The model under review builds one solid part; all positions refer to its coordinate system, in mm. Round coordinates to 2 decimals unless told otherwise and drop trailing zeros. Loops run counter-clockwise (first coordinate to the right, second up) from the corner with the lowest first, then second, coordinate; pieces in that order, holes last. Notation, with made-up numbers: M 11,21 L 56,21 A22 ccw 56,29 Z; hole C 36,68 d11. An arc over 180 degrees is marked long. Answer in a Markdown table with one row per item. Add a question column.
Autodesk Inventor part; units mm, degrees
ref_plane "YZ Plane" through (0, 0, 0) normal (1, 0, 0) x (0, 1, 0)
ref_plane "XZ Plane" through (0, 0, 0) normal (0, 1, 0) x (-1, 0, 0)
ref_plane "XY Plane" through (0, 0, 0) normal (0, 0, 1) x (1, 0, 0)
sketch "Sketch1" plane through (0, 0, 0) normal (0, 0, 1) x (1, 0, 0)
  circle A0 centre (0, 0) radius 47.625
  dimension "d0" = 95.25
extrude "Extrusion1" add sketch "Sketch1" along normal blind 3.175
sketch "Sketch4" plane through (0, 0, 3.175) normal (0, 0, 1) x (1, 0, 0)
  circle A0 centre (12.446, -29.7561) radius 3.3655
  point P0 (0, 0)
  dimension "d16" = 6.731
  dimension "d17" = 12.446
  dimension "d18" = 29.7561
extrude "Extrusion4" cut sketch "Sketch4" against normal blind 3.175
sketch "Sketch6" plane through (0, 0, 3.175) normal (0, 0, 1) x (1, 0, 0)
  circle A0 centre (0, 0) radius 3.3655
  circle A1 centre (0, 0) radius 9.525
  circle A2 centre (0, 0) radius 47.625
  circle A3 centre (12.446, -29.7561) radius 3.3655
  line L0 (0, 0) -> (12.446, -29.7561) construction
  dimension "d32" = 6.731
  dimension "d33" = 19.05
  dimension "d191" = 32.2541
extrude "Extrusion7" add sketch "Sketch6" along normal blind 3.81 contours A1
sketch "Sketch7" plane through (0, 0, 3.175) normal (0, 0, 1) x (1, 0, 0)
  line L0 (0, 0) -> (21.4313, 37.12)
  line L1 (0, 0) -> (42.8625, 0) construction
  circle A0 centre (21.4313, 37.12) radius 1.8415
  circle A1 centre (-21.4312, 37.12) radius 1.8415
  circle A2 centre (-42.8625, 0) radius 1.8415
  circle A3 centre (-21.4313, -37.12) radius 1.8415
  circle A4 centre (21.4312, -37.12) radius 1.8415
  circle A5 centre (42.8625, 0) radius 1.8415
  dimension "d39" = 42.8625
  dimension "d40" = 60
  dimension "d41" = 3.683
  dimension "d44" = 360
extrude "Extrusion10" cut sketch "Sketch7" against normal through all
sketch "Sketch9" plane through (0, 0, 3.175) normal (0, 0, 1) x (1, 0, 0)
  circle A0 centre (0, 0) radius 3.3655
  line L0 (0, 0) -> (0, 41.91)
  circle A1 centre (0, 41.91) radius 1.8415
  circle A2 centre (-36.2951, 20.955) radius 1.8415
  circle A3 centre (-36.2951, -20.955) radius 1.8415
  circle A4 centre (0, -41.91) radius 1.8415
  circle A5 centre (36.2951, -20.955) radius 1.8415
  circle A6 centre (36.2951, 20.955) radius 1.8415
  dimension "d61" = 41.91
  dimension "d62" = 3.683
  dimension "d65" = 360
extrude "Extrusion12" cut sketch "Sketch9" against normal blind 25.4 contours A1 | A2 | A3 | A4 | A5 | A6
sketch "Sketch17" plane through (0, 0, 3.175) normal (0, 0, 1) x (1, 0, 0)
  line L0 (0, 0) -> (39.3779, 10.5513)
  line L1 (0, 0) -> (40.767, 0) construction
  circle A0 centre (39.3779, 10.5513) radius 2.794
  line L2 (0, 0) -> (0, 17.3134)
  circle A1 centre (39.3779, -10.5513) radius 2.794
  circle A2 centre (-39.3779, 10.5513) radius 2.794
  circle A3 centre (-39.3779, -10.5513) radius 2.794
  line L3 (0, 0) -> (28.8266, 28.8266)
  line L4 (0, 0) -> (40.767, 0) construction
  circle A4 centre (28.8266, 28.8266) radius 2.794
  circle A5 centre (-28.8266, 28.8266) radius 2.794
  dimension "d144" = 40.767
  dimension "d145" = 15
  dimension "d146" = 5.588
  dimension "d149" = 40.767
  dimension "d150" = 45
  dimension "d151" = 5.588
extrude "Extrusion22" cut sketch "Sketch17" against normal blind 25.4 contours A0 | A1 | A2 | A3
extrude "Extrusion23" cut sketch "Sketch17" against normal blind 25.4 contours A4 | A5
sketch "Sketch22" plane through (0, 0, 3.175) normal (0, 0, 1) x (1, 0, 0)
  circle A0 centre (-7.9375, 29.1338) radius 3.3655
  point P0 (0, 0)
  dimension "d166" = 6.731
  dimension "d167" = 7.9375
  dimension "d168" = 29.1338
extrude "Extrusion26" cut sketch "Sketch22" against normal through all
sketch "Sketch23" plane through (0, 0, 3.175) normal (0, 0, 1) x (1, 0, 0)
  circle A0 centre (0, 0) radius 3.3655
extrude "Extrusion27" cut sketch "Sketch23" against normal blind 1.5875
chamfer "Chamfer6" distance 3.175 angle 45 1 edges at (-9.525, 0, 6.985)
sketch "Sketch24" plane through (0, 0, 3.175) normal (0, 0, 1) x (1, 0, 0)
  circle A0 centre (12.446, -29.7561) radius 3.3655
  circle A1 centre (12.446, -29.7561) radius 5.715
  point P0 (0, 0)
  dimension "d176" = 11.43
extrude "Extrusion28" add sketch "Sketch24" along normal blind 3.175
sketch "Sketch25" plane through (0, 0, 0) normal (0, 0, -1) x (-1, 0, 0)
  circle A0 centre (-12.446, -29.7561) radius 3.3655
  circle A1 centre (-12.446, -29.7561) radius 1.905
  point P0 (0, 0)
  dimension "d179" = 3.81
extrude "Extrusion29" add sketch "Sketch25" against normal blind 3.175
fillet "Fillet3" radius 1.27 1 edges at (6.731, -29.7561, 3.175)
sketch "Sketch26" plane through (0, 0, 3.175) normal (0, 0, 1) x (1, 0, 0)
  circle A0 centre (-7.9375, 38.862) radius 3.3655
  circle A1 centre (7.9375, 38.862) radius 1.905
  line L0 (7.9375, 38.862) -> (-7.9375, 38.862) construction
  circle A2 centre (-7.9375, 29.1338) radius 3.3655 construction
  line L1 (-7.9375, 29.1338) -> (-7.9375, 38.862) construction
  point P0 (0, 0)
  point P1 (0, 38.862)
  dimension "d183" = 6.731
  dimension "d184" = 3.81
  dimension "d185" = 38.862
  dimension "d186" = 15.875
  dimension "d189" = 9.7282
extrude "Extrusion30" cut sketch "Sketch26" against normal through all
sketch "Sketch27" plane through (0, 0, 3.175) normal (0, 0, 1) x (1, 0, 0)
  line L0 (-24.0461, 24.2224) -> (-19.7824, 24.2224) construction
  line L1 (-19.7824, 24.2224) -> (-19.7824, 20.2457) construction
  line L2 (-19.7824, 20.2457) -> (-24.0461, 20.2457) construction
  line L3 (-24.0461, 20.2457) -> (-24.0461, 24.2224) construction
  line L4 (25.5336, -15.2981) -> (30.1056, -15.2981) construction
  line L5 (30.1056, -15.2981) -> (30.1056, -17.0126) construction
  line L6 (30.1056, -17.0126) -> (25.5336, -17.0126) construction
  line L7 (25.5336, -17.0126) -> (25.5336, -15.2981) construction
sketch "Sketch29" plane through (0, 0, 3.175) normal (0, 0, 1) x (1, 0, 0)
  circle A0 centre (0, 41.91) radius 1.8415
  circle A1 centre (0, 41.91) radius 3.683
  point P0 (0, 0)
  dimension "d192" = 7.366
extrude "Extrusion31" cut sketch "Sketch29" against normal blind 1.27
pattern_circular "Circular Pattern1" count 6 over 360 about axis through (0, 0, 0) along (0, 0, 1) of "Extrusion31"
sketch "Sketch21" plane through (0, 0, 0) normal (0, 0, -1) x (-1, 0, 0)
  circle A0 centre (0, 0) radius 47.625
  circle A1 centre (0, 0) radius 9.525
  circle A2 centre (0, 0) radius 47.1805
  dimension "d162" = 95.25
  dimension "d163" = 94.361
extrude "PRINT_FEATURE_1" [suppressed]
properties part number "aftSpoolSectionSealingWall" material "ABS Plastic"
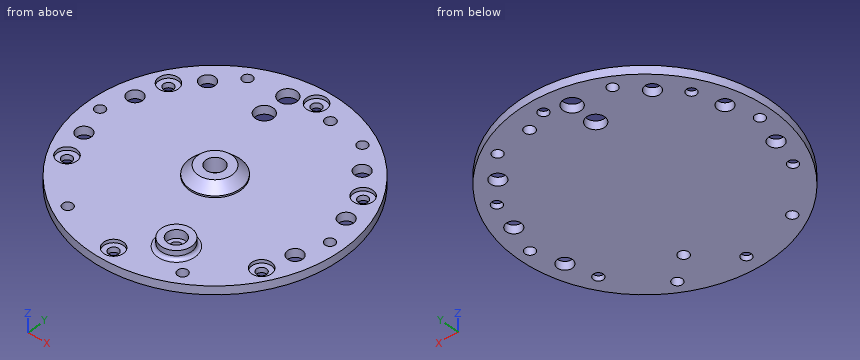
1. For pin 1 Ø6 at (x, y) = (12.45, -29.76) entering from +Z (3 decimals); pin 2 Ø5 at (x, y) = (-36.3, -20.96) entering from +Z (3 decimals); pin 3 Ø4.5 at (x, y) = (-39.38, 10.55) entering from +Z; pin 4 Ø7.5 at (x, y) = (12.5, -30) entering from +Z, all flat-tipped, find the tip position at first contact; note any pin that passes through.
2. To check wall thickness, follow probe 1 along X at (y, z) = (21, 3); probe 2 along X at (y, z) = (-13, 1.25); probe 3 along Z at (x, y) = (9.5, -29) (3 decimals). State the ranges of each line that lie inside material, in increasing order.
3. Take a section at A-A, the plane y = 0. State how many separate pieces and enclosed holes the cut face has, and give its area (3 significant figures).
4. Take a section at C-C, the plane y = -41.91. State the section outline as (x, z) points (1 decimal), and give its area (3 significant figures).
Check sheet entries:
| question | item | result |
|---|---|---|
| 1 | pin 1 | stops at z = 3.175 |
| 1 | pin 2 | stops at z = 1.905 |
| 1 | pin 3 | passes through |
| 1 | pin 4 | stops at z = 6.35 |
| 2 | probe 1 | x = -42.75 to -39.98, -32.61 to 32.61, 39.98 to 42.75 |
| 2 | probe 2 | x = -45.82 to -40.72, -38.03 to 38.03, 40.72 to 45.82 |
| 2 | probe 3 | z = 0 to 3.175 |
| 3 | separate pieces | 3 |
| 3 | enclosed holes | 0 |
| 3 | area | 305 mm^2 |
| 4 | outline | M -22.6,0 L -1.8,0 L -1.8,1.9 L -3.7,1.9 L -3.7,3.2 L -22.6,3.2 Z; M 1.8,0 L 22.6,0 L 22.6,3.2 L 3.7,3.2 L 3.7,1.9 L 1.8,1.9 Z |
| 4 | area | 127 mm^2 |
